The listing builds one solid part. Answer for the finished solid, in the listing's coordinates (mm). Face numbers are marked on the shaded views. A direction names the side the tool comes from. Round coordinates to 2 decimals unless told otherwise and drop trailing zeros. Order: outer loops, then holes, each group sorted by start corner. A loop starts at its lowest first (then second) coordinate and runs counter-clockwise, first axis right, second up. Notation, with made-up numbers: M 78.25,-36 L 136.25,-36 A29 cw 136.25,-11 Z; hole C -19,-10.5 d3. An arc over 180 degrees is marked long. Write item = value, one per line. Start each with the question number.
(1) A cutting plane is placed at C-C, the plane y = -15.5. Determine the outline of the cut face in (x, z).
(2) Straight lines are drawn through the part: probe 1 along Y at (x, z) = (0.5, 6.5); probe 2 along Y at (x, z) = (2, 3.5); probe 3 along Z at (x, y) = (4.25, -9). For each, find the intervals that lie inside material, in ascending order. Write a range as from..to.
(3) Which of the six approach directions +Z, -Z, +X, -X, +Y, -Y give full straight-line access (tool end or side, diameter ignored) to the marked faces 5, 6 and 7?
(4) Each of these flat-tipped pins is pushed along its axis until it touches: pin 1 (1.8 mm diameter, centred on x = 0, z = 2.5, fed in from +Y); pin 2 (1 mm diameter, centred on x = -4.5, y = 3, fed in from +Z); pin 3 (10 mm diameter, centred on x = 7, y = 4.5, fed in from +Z). Where does it stop, or does it pass through?
(5) A cutting plane is placed at A-A, the plane y = 0.5. Determine the outline of the cut face in (x, z).
(6) A cutting plane is placed at B-B, the plane y = -6. Determine the outline of the cut face in (x, z).
(7) For a pull along Y with two mould halves and no side action, classify the marked faces 1, 2, 3 and 4 as released by +Y, released by -Y, zero draft, split by the parting line, or undercut.
from build123d import *

# Parameters (mm, degrees)
SKETCH_1_R          = 6.35
EXTRUDE_1_DEPTH     = 9.6
SKETCH_2_R          = 7.125
EXTRUDE_2_DEPTH     = 1
SKETCH_3_R          = 6.25
EXTRUDE_3_DEPTH     = 12.38
SKETCH_4_R          = 6.85
EXTRUDE_4_DEPTH     = 6
CHAMFER_1_SIZE      = 1.7
SKETCH_5_R          = 5.25
EXTRUDE_5_DEPTH     = 7
SKETCH_6_R          = 9
EXTRUDE_6_DEPTH     = 1
SKETCH_7_R          = 9
SKETCH_7_R_2        = 8
EXTRUDE_7_DEPTH     = 5
FILLET_1_R          = 2
SKETCH_8_R          = 1
EXTRUDE_8_DEPTH     = 2
SKETCH_9_R          = 1.5
CUT_EXTRUDE_1_DEPTH = 9.6
SKETCH_10_R         = 1
CUT_EXTRUDE_2_DEPTH = 0.1


with BuildPart() as part:
    # 草图1 → 凸台-拉伸1 (new body)
    with BuildSketch(Plane(origin=(0, 0, 0), x_dir=(1, 0, 0), z_dir=(0, 1, 0))):
        with Locations(Location((0, 0, 0), (0, 0, 270))):
            Circle(SKETCH_1_R)
    extrude(amount=EXTRUDE_1_DEPTH)

    # 草图2 → 凸台-拉伸2 (add)
    with BuildSketch(Plane(origin=(0, 0, 0), x_dir=(-1, 0, 0), z_dir=(0, -1, 0))):
        with Locations(Location((0, 0, 0), (0, 0, 90))):
            Circle(SKETCH_2_R)
    extrude(amount=EXTRUDE_2_DEPTH)

    # 草图3 → 凸台-拉伸3 (add)
    with BuildSketch(Plane.XZ.offset(1)):
        with Locations(Location((0, 0, 0), (0, 0, 270))):
            Circle(SKETCH_3_R)
    extrude(amount=EXTRUDE_3_DEPTH)

    # 草图4 → 凸台-拉伸4 (add)
    with BuildSketch(Plane.XZ.offset(13.38)):
        with Locations(Location((0, 0, 0), (0, 0, 270))):
            Circle(SKETCH_4_R)
    extrude(amount=EXTRUDE_4_DEPTH)

    # 倒角1
    chamfer_1_edges = [part.edges().sort_by_distance(p)[0] for p in [
        (0, -19.38, 6.85),
    ]]
    chamfer(chamfer_1_edges, length=CHAMFER_1_SIZE)

    # 草图5 → 凸台-拉伸5 (add)
    with BuildSketch(Plane.XZ.offset(19.38)):
        with Locations(Location((0, 0, 0), (0, 0, 270))):
            Circle(SKETCH_5_R)
    extrude(amount=EXTRUDE_5_DEPTH)

    # 草图6 → 凸台-拉伸6 (add)
    with BuildSketch(Plane(origin=(0, -5, 0), x_dir=(-1, 0, 0), z_dir=(0, -1, 0))):
        with Locations(Location((0, 0, 0), (0, 0, 90))):
            Circle(SKETCH_6_R)
    extrude(amount=-EXTRUDE_6_DEPTH)

    # 草图7 → 凸台-拉伸7 (add)
    with BuildSketch(Plane(origin=(0, -4, 0), x_dir=(1, 0, 0), z_dir=(0, 1, 0))):
        with Locations(Location((0, 0, 0), (0, 0, 90))):
            Circle(SKETCH_7_R)
        with Locations(Location((0, 0, 0), (0, 0, 270))):
            Circle(SKETCH_7_R_2, mode=Mode.SUBTRACT)
    extrude(amount=EXTRUDE_7_DEPTH)

    # 圆角1
    # the kernel refuses this fillet: 2 mm, written as the material it adds along each edge
    with BuildSketch(Plane(origin=(0, -4, 0), x_dir=(0, 0, 1), z_dir=(-1, 0, 0))) as fillet_1_piece_1:
        with BuildLine():
            CenterArc((6, 1.984313483), FILLET_1_R, 277.180755781, 82.819244219)
            Line((6.25, 0), (8, 0))
            Line((8, 0), (8, 1.984313483))
        make_face()
    revolve(axis=Axis((0, -4, 0), (0, 1, 0)))
    # the kernel refuses this fillet: 2 mm, written as the material it takes off along each edge
    with BuildSketch(Plane(origin=(0, -5, 0), x_dir=(0, 0, -1), z_dir=(-1, 0, 0))) as fillet_1_2_piece_1:
        with BuildLine():
            CenterArc((9 - FILLET_1_R, -FILLET_1_R), FILLET_1_R, 0, 90)
            Line((9, -FILLET_1_R), (9, 0))
            Line((9, 0), (9 - FILLET_1_R, 0))
        make_face()
    revolve(axis=Axis((0, -5, 0), (0, -1, 0)), mode=Mode.SUBTRACT)

    # 草图8 → 凸台-拉伸8 (add)
    with BuildSketch(Plane.XZ.offset(26.38)):
        with Locations(Location((0, -2.5, 0), (0, 0, 270))):
            Circle(SKETCH_8_R)
        with Locations(Location((0, 2.5, 0), (0, 0, 270))):
            Circle(SKETCH_8_R)
    extrude(amount=EXTRUDE_8_DEPTH)

    # 草图9 → 切除-拉伸1 (cut)
    with BuildSketch(Plane(origin=(0, 9.6, 0), x_dir=(1, 0, 0), z_dir=(0, 1, 0))):
        with Locations((-6.35, 0)):
            Circle(SKETCH_9_R)
    extrude(amount=-CUT_EXTRUDE_1_DEPTH, mode=Mode.SUBTRACT)

    # 草图10 → 切除-拉伸2 (cut)
    with BuildSketch(Plane(origin=(0, 9.6, 0), x_dir=(1, 0, 0), z_dir=(0, 1, 0))):
        with Locations(Location((0, -2.5, 0), (0, 0, 90))):
            Circle(SKETCH_10_R)
        with Locations(Location((0, 2.5, 0), (0, 0, 90))):
            Circle(SKETCH_10_R)
    extrude(amount=-CUT_EXTRUDE_2_DEPTH, mode=Mode.SUBTRACT)


solid = part.part
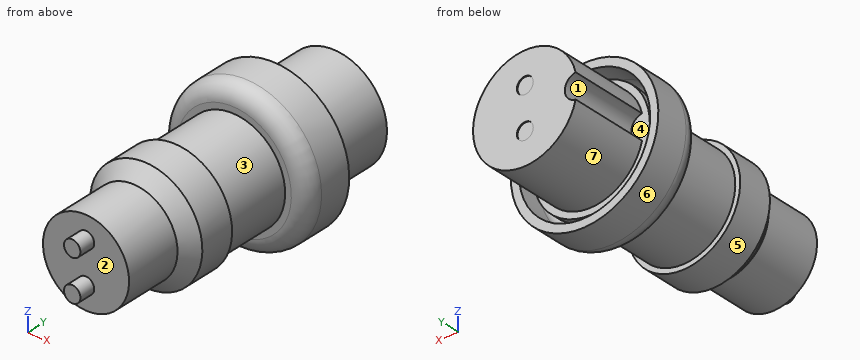
Reported:
q1.outline = C 0,0 d13.7
q2.probe_1 = -18.01..-13.38, -5..-3.95, -1..0
q2.probe_2 = -26.38..9.6
q2.probe_3 = -4.58..4.58
q3.face_5 = -Y
q3.face_6 = +Y, -Y
q3.face_7 = +Y
q4.pin_1 = 9.5
q4.pin_2 = 4.93
q4.pin_3 = 8.32
q5.outline = C 0,0 d18; M -6.17,-1.49 A6.35 ccw long -6.17,1.49 A1.5 cw Z; hole C 0,0 d16
q6.outline = C 0,0 d12.5
q7.face_1 = zero draft
q7.face_2 = released by -Y
q7.face_3 = undercut
q7.face_4 = released by +Y
